```python
from build123d import *

# Parameters (mm, degrees)
SKETCH1_W           = 60.325
SKETCH1_H           = 12.7
SKETCH1_R           = 2.159
BOSS_EXTRUDE1_DEPTH = 12.7
SKETCH4_W           = 43.775259309
SKETCH4_H           = 12.7
BOSS_EXTRUDE2_DEPTH = 3.175
SKETCH5_R           = 3.556
CUT_EXTRUDE1_DEPTH  = 3.81
FILLET5_R           = 0.762


with BuildPart() as part:
    # Sketch1 → Boss-Extrude1 (new body)
    with BuildSketch(Plane(origin=(0, 0, 0), x_dir=(1, 0, 0), z_dir=(0, 1, 0))):
        with Locations((30.1625, 6.35)):
            Rectangle(SKETCH1_W, SKETCH1_H)
        with Locations((17.4625, 6.35)):
            Circle(SKETCH1_R, mode=Mode.SUBTRACT)
        with Locations((42.8625, 6.35)):
            Circle(SKETCH1_R, mode=Mode.SUBTRACT)
    extrude(amount=BOSS_EXTRUDE1_DEPTH)

    # Sketch4 → Boss-Extrude2 (add)
    with BuildSketch(Plane.ZY):
        with Locations((-21.887629655, 6.35)):
            Rectangle(SKETCH4_W, SKETCH4_H)
    extrude(amount=BOSS_EXTRUDE2_DEPTH)

    # Sketch5 → Cut-Extrude1 (cut)
    with BuildSketch(Plane.XZ):
        with Locations((42.8625, -6.35)):
            Circle(SKETCH5_R)
        with Locations((17.4625, -6.35)):
            Circle(SKETCH5_R)
    extrude(amount=-CUT_EXTRUDE1_DEPTH, mode=Mode.SUBTRACT)

    # Fillet5
    fillet5_edges = [part.edges().sort_by_distance(p)[0] for p in [
        (60.325, 12.7, -6.35),
        (30.1625, 12.7, -12.7),
        (0, 6.35, -43.775259309),
        (-1.5875, 12.7, -43.775259309),
        (0, 0, -28.237629654),
        (-1.5875, 0, -43.775259309),
        (0, 12.7, -28.237629654),
        (-3.175, 6.35, -43.775259309),
        (-3.175, 0, -21.887629654),
        (-3.175, 6.35, 0),
        (-3.175, 12.7, -21.887629654),
        (39.3065, 0, -6.35),
        (13.9065, 0, -6.35),
        (30.1625, 0, -12.7),
        (60.325, 0, -6.35),
        (28.575, 0, 0),
        (28.575, 12.7, 0),
        (60.325, 6.35, -12.7),
        (60.325, 6.35, 0),
    ]]
    fillet(fillet5_edges, radius=FILLET5_R)


solid = part.part
```
Work out the finished part from the listing and answer in its coordinate system (mm). A direction names the side the tool comes from. Round coordinates to 2 decimals unless told otherwise and drop trailing zeros. Write each loop counter-clockwise with the first axis right and the second up, starting at its lowest first coordinate (ties: lowest second). Pieces come first, ordered by that corner, then holes.
1) Consider probe 1 along X at (y, z) = (6.75, -6.35) (1 decimal); probe 2 along X at (y, z) = (4, -17.5) (3 decimals); probe 3 along Z at (x, y) = (4.5, 5.75). Determine where each line is inside the solid, lowest interval first.
2) Which of the six approach directions +Z, -Z, +X, -X, +Y, -Y give full straight-line access (tool end or side, diameter ignored) to faces 4 (the face through (24, 0, -9)), 5 (the face through (45.2, 3.81, -6.3)), 6 (the face through (0, 6, -28))?
3) A cutting plane is placed at C-C on x = 33. Determine the outline of the cut face in (y, z).
4) A cutting plane is placed at A-A on y = 2.5. Give the number of separate pieces and of enclosed holes in the cut face, and give its area (3 significant figures).
5) A cutting plane is placed at B-B on z = -6.35. Determine the outline of the cut face in (x, y) (1 decimal), and give its area (3 significant figures).
6) A cutting plane is placed at D-D on z = -34.5. Determine the outline of the cut face in (x, y) (3 decimals), and give its area (3 significant figures).
7) Flat-ended cylindrical pins translate along their axes: P1, Ø5.5, axis at x = 18.5, z = -6, coming from the -Y side; P2, Ø5, axis at y = 9.5, z = -29, coming from the +X side. Find the tip coordinate at first contact, or state that the pin passes through.
8) Determine the mould class of faces 1 (the face through (60.325, 6, -6)), 2 (the face through (44.857, 8.193, -5.523)), 3 (the face through (-3.175, 6, -22)) for opening direction X: pulls with the +X half, pulls with the -X half, needs draft (parallel to the pull), parting line crosses it, or undercut.
Entries:
1. probe 1: x = -3.2 to 15.3, 19.6 to 40.7, 45 to 60.3
1. probe 2: x = -3.175 to 0
1. probe 3: z = -12.7 to 0
2. face 4: +Z, -Z, +X, -X, -Y
2. face 5: -Y
2. face 6: -Z, +X, +Y, -Y
3. outline: (0, -11.94) arc R0.76 ccw to (0.76, -12.7) - (11.94, -12.7) arc R0.76 ccw to (12.7, -11.94) - (12.7, -0.76) arc R0.76 ccw to (11.94, 0) - (0.76, 0) arc R0.76 ccw to (0, -0.76) - close
4. separate pieces: 1
4. enclosed holes: 2
4. area: 825 mm2
5. outline: (-3.2, 0.8) arc R0.8 ccw to (-2.4, 0) - (13.1, 0) arc R0.8 ccw to (13.9, 0.8) - (13.9, 3.8) - (15.3, 3.8) - (15.3, 12.7) - (-2.4, 12.7) arc R0.8 ccw to (-3.2, 11.9) - close; (19.6, 3.8) - (21, 3.8) - (21, 0.8) arc R0.8 ccw to (21.8, 0) - (38.5, 0) arc R0.8 ccw to (39.3, 0.8) - (39.3, 3.8) - (40.7, 3.8) - (40.7, 12.7) - (19.6, 12.7) - close; (45, 3.8) - (46.4, 3.8) - (46.4, 0.8) arc R0.8 ccw to (47.2, 0) - (59.6, 0) arc R0.8 ccw to (60.3, 0.8) - (60.3, 11.9) arc R0.8 ccw to (59.6, 12.7) - (45, 12.7) - close
5. area: 674 mm2
6. outline: (-3.175, 0.762) arc R0.762 ccw to (-2.413, 0) - (-0.762, 0) arc R0.762 ccw to (0, 0.762) - (0, 11.938) arc R0.762 ccw to (-0.762, 12.7) - (-2.413, 12.7) arc R0.762 ccw to (-3.175, 11.938) - close
6. area: 39.8 mm2
7. P1: stops at y = 0.16
7. P2: stops at x = 0
8. face 1: pulls with the +X half
8. face 2: undercut
8. face 3: pulls with the -X half
